Verification items for the finished model (mm, model axes). A direction names the side the tool comes from. Round coordinates to 2 decimals unless told otherwise and drop trailing zeros. Order: outer loops, then holes, each group sorted by start corner. A loop starts at its lowest first (then second) coordinate and runs counter-clockwise, first axis right, second up. Notation, with made-up numbers: M -16,74.5 L 41,74.5 A17 ccw 41,86.5 Z; hole C -19.5,-37 d9. An arc over 180 degrees is marked long. Answer as a JSON object with one key per item and string values. Group by question number.
```python
from build123d import *

# Parameters (mm, degrees)
SKETCH1_W           = 150
SKETCH1_H           = 90
BOSS_EXTRUDE1_DEPTH = 55
SHELL4_T            = -5
SKETCH2_R           = 20
BOSS_EXTRUDE2_DEPTH = 2.5
SKETCH3_R           = 7.5
BOSS_EXTRUDE3_DEPTH = 50
SKETCH4_W           = 65
SKETCH4_H           = 19.658499389
CUT_EXTRUDE1_DEPTH  = 185.136498283
SKETCH6_W           = 3
SKETCH6_H           = 3
CUT_EXTRUDE3_DEPTH  = 40
FILLET4_R           = 5
FILLET5_R           = 5
SKETCH10_W          = 3
SKETCH10_H          = 3
CUT_EXTRUDE4_DEPTH  = 40


with BuildPart() as part:
    # Sketch1 → Boss-Extrude1 (new body)
    with BuildSketch(Plane.XY):
        with Locations((75, -45)):
            Rectangle(SKETCH1_W, SKETCH1_H)
    extrude(amount=BOSS_EXTRUDE1_DEPTH)

    # Shell4
    shell4_openings = [part.faces().sort_by_distance(p)[0] for p in [
        (75, -45, 55),
    ]]
    offset(amount=SHELL4_T, openings=shell4_openings, kind=Kind.INTERSECTION)

    # Sketch2 → Boss-Extrude2 (add)
    with BuildSketch(Plane.XY.offset(5)):
        with Locations((45, -45)):
            Circle(SKETCH2_R)
        with Locations((105, -45)):
            Circle(SKETCH2_R)
    extrude(amount=BOSS_EXTRUDE2_DEPTH)

    # Sketch3 → Boss-Extrude3 (add)
    with BuildSketch(Plane.XY.offset(7.5)):
        with Locations((45, -45)):
            Circle(SKETCH3_R)
        with Locations((105, -45)):
            Circle(SKETCH3_R)
    extrude(amount=BOSS_EXTRUDE3_DEPTH)

    # Sketch4 → Cut-Extrude1 (cut, through all)
    with BuildSketch(Plane.XZ.offset(90)):
        Polygon((85, 55), (85, 49.954434269), (85, 34.954434269), (150, 34.954434269), (150, 55), align=None)
        with Locations((117.5, 64.829249694)):
            Rectangle(SKETCH4_W, SKETCH4_H)
    extrude(amount=-CUT_EXTRUDE1_DEPTH, mode=Mode.SUBTRACT)

    # Sketch6 → Cut-Extrude3 (cut)
    with BuildSketch(Plane.XY.offset(34.954434269)):
        with Locations((96.5, -2.5)):
            Rectangle(SKETCH6_W, SKETCH6_H)
        with Locations((113.5, -2.5)):
            Rectangle(SKETCH6_W, SKETCH6_H)
        with Locations((96.5, -87.5)):
            Rectangle(SKETCH6_W, SKETCH6_H)
        with Locations((113.5, -87.5)):
            Rectangle(SKETCH6_W, SKETCH6_H)
    extrude(amount=-CUT_EXTRUDE3_DEPTH, mode=Mode.SUBTRACT)

    # Fillet4
    fillet4_edges = [part.edges().sort_by_distance(p)[0] for p in [
        (5, -5, 30),
        (5, -85, 30),
        (145, -5, 19.977217134),
        (145, -85, 19.977217134),
        (150, 0, 17.477217134),
        (150, -90, 17.477217134),
        (85, -87.5, 55),
        (85, -87.5, 34.954434269),
        (85, -2.5, 55),
        (85, -2.5, 34.954434269),
        (0, 0, 27.5),
        (0, -90, 27.5),
    ]]
    fillet(fillet4_edges, radius=FILLET4_R)

    # Fillet5
    fillet5_edges = [part.edges().sort_by_distance(p)[0] for p in [
        (37.5, -45, 57.5),
        (97.5, -45, 34.954434269),
    ]]
    fillet(fillet5_edges, radius=FILLET5_R)

    # Sketch10 → Cut-Extrude4 (cut)
    with BuildSketch(Plane.XY.offset(55)):
        with Locations((2.5, -45)):
            Rectangle(SKETCH10_W, SKETCH10_H)
        with Locations((37.5, -87.5)):
            Rectangle(SKETCH10_W, SKETCH10_H)
        with Locations((37.5, -2.5)):
            Rectangle(SKETCH10_W, SKETCH10_H)
    extrude(amount=-CUT_EXTRUDE4_DEPTH, mode=Mode.SUBTRACT)


solid = part.part
```
Q1. Thickness scan on line 1 (X direction, y = -31, z = 10); line 2 (Y direction, x = 77.5, z = 17.5); line 3 (Z direction, x = 20, y = -61.5). Record the ranges inside material, lowest first. Write a range as from..to.
Q2. Cross-section at C-C, the plane y = -75.5. Record the cut outline in (x, z).
Q3. Cross-section at D-D, the plane x = 121. Record the cut outline in (y, z).
Q4. Gauge pin test, flat ends, axial feed: pin 1 Ø0.9 at (x, y) = (37, -3) entering from +Z; pin 2 Ø0.9 at (y, z) = (-2, 40) entering from +X; pin 3 Ø1 at (x, y) = (34, -43.5) entering from +Z. Record the tip position at first contact, or that the pin passes through.
Q5. Release check for a two-part mould opening along Y. For faces 1 (the face through (36, -3, 35)), 2 (the face through (0, -46, 27)) record: released by +Y, released by -Y, zero draft, split by the parting line, or undercut.
Q6. Cross-section at A-A, the plane z = 12. Give the number of separate pieces and of enclosed holes in the cut face, then the cut area to 3 significant figures.
Q7. Tool access check on faces 3 (the face through (6, -83, 30)), 4 (the face through (74, -44, 0)), 5 (the face through (147, -55, 34.954)), 6 (the face through (112, -3, 18)). Record the directions out of +Z, -Z, +X, -X, +Y, -Y that give a thin tool (end or side, any length) a straight path to the whole face; none if there is none.
Conclusion:
{
 "1": {"line 1": "0..5, 145..150", "line 2": "-90..-85, -5..0", "line 3": "0..5"},
 "2": {"outline": "M 0,0 L 150,0 L 150,34.95 L 145,34.95 L 145,5 L 5,5 L 5,55 L 0,55 Z"},
 "3": {"outline": "M -90,0 L 0,0 L 0,34.95 L -5,34.95 L -5,5 L -33,5 L -33,7.5 L -57,7.5 L -57,5 L -85,5 L -85,34.95 L -90,34.95 Z"},
 "4": {"pin 1": "z = 15", "pin 2": "x = 85.02", "pin 3": "z = 7.5"},
 "5": {"face 1": "undercut", "face 2": "zero draft"},
 "6": {"separate pieces": "3", "enclosed holes": "5", "area": "2,620 mm2"},
 "7": {"face 3": "+Z", "face 4": "-Z, +X, -X, +Y, -Y", "face 5": "+Z, +X, +Y, -Y", "face 6": "+Z, -Z"}
}
